Read the model definition and answer for the solid it produces. Units are mm, in the model's axes. A direction names the side the tool comes from. Coordinates: 2 decimals unless noted, no trailing zeros. Order: outer loops, then holes, each group sorted by start corner. A loop starts at its lowest first (then second) coordinate and runs counter-clockwise, first axis right, second up. Notation, with made-up numbers: (-6.5, -22) - (9.5, -22) arc R25 cw to (9.5, 6) - close; hole circle Ø11 at (-12, 2). An arc over 180 degrees is marked (long way). Use one line per item in the form item = value.
Autodesk Inventor part; units mm, degrees
ref_plane "YZ Plane" through (0, 0, 0) normal (1, 0, 0) x (0, 1, 0)
ref_plane "XZ Plane" through (0, 0, 0) normal (0, 1, 0) x (-1, 0, 0)
ref_plane "XY Plane" through (0, 0, 0) normal (0, 0, 1) x (1, 0, 0)
sketch "스케치6" plane through (0, 0, 0) normal (0, 1, 0) x (-1, 0, 0)
  circle A0 centre (0, 0) radius 15
  dimension "d16" = 30
extrude "돌출4" add sketch "스케치6" along normal blind 1.5
sketch "스케치7" plane through (0, 1.5, 0) normal (0, 1, 0) x (1, 0, 0)
  circle A0 centre (0, 0) radius 15
  arc A1 (0, 0) -> (-15, 0) centre (-7.5, -6.6144) ccw
  arc A2 (0, 0) -> (0, 15) centre (-6.6144, 7.5) ccw
  arc A3 (0, 0) -> (15, 0) centre (7.5, 6.6144) ccw
  arc A4 (0, 0) -> (0, -15) centre (6.6144, -7.5) ccw
  line L0 (0, -15) -> (0, 0)
  line L1 (0, 0) -> (15, 0)
  line L2 (0, 0) -> (0, 15)
  line L3 (0, 0) -> (-15, 0)
  arc A5 (-15, 0) -> (0, -15) centre (0, 0) ccw
  arc A6 (0, -15) -> (15, 0) centre (0, 0) ccw
  arc A7 (15, 0) -> (0, 15) centre (0, 0) ccw
  arc A8 (0, 15) -> (-15, 0) centre (0, 0) ccw
  point P0 (0, -15)
  point P1 (0, -15)
  dimension "d19" = 10
  dimension "d20" = 10
  dimension "d21" = 10
  dimension "d22" = 10
  dimension "d23" = 15
  dimension "d24" = 15
extrude "돌출5" cut sketch "스케치7" against normal blind 1.5 contours L1 A2 A0 | A0 L0 A3 | L2 A1 A0 | A0 L3 A4
sketch "스케치8" plane through (0, 1.5, 0) normal (0, 1, 0) x (1, 0, 0)
  arc A0 (0, 0) -> (0, -15) centre (6.6144, -7.5) ccw
  circle A1 centre (0, 0) radius 0.75
  dimension "d27" = 1.5
extrude "돌출6" add sketch "스케치8" against normal blind 1.5
sketch "스케치9" plane through (0, 1.5, 0) normal (0, 1, 0) x (1, 0, 0)
  point P0 (0, 0)
properties part number "fan_num4_1"
(1) Given pin 1 Ø0.8 at (x, y) = (6.5, 0.5) entering from -Z; pin 2 Ø0.8 at (y, z) = (1, 9) entering from +X, each flat-ended and moving along its own axis, determine where each tip first touches the part or whether it passes through.
Answer list:
pin_1 = 0
pin_2 = 0
(2) The mould has two halves that part along Z. Classify faces 5 (the cylindrical face through (-3.382, 0.76, 7.762)), 6 (the cylindrical face through (7.762, 0.76, 3.382)), 7 (the flat face through (0, 0, 0)): +Z half, -Z half, draft (parallel to the pull), parting line (faces both ways), or undercut.
Answer list:
face_5 = undercut
face_6 = +Z half
face_7 = draft
(3) Section B-B, the plane z = 1.25 is taken. Write down the section's boundary in (x, y).
Answer list:
outline = (-1.19, 0) - (0, 0) - (0, 1.5) - (-1.19, 1.5) - close; (1.32, 0) - (13.68, 0) - (13.68, 1.5) - (1.32, 1.5) - close
(4) Straight lines are drawn through the part: L1, parallel to Z at x = -1.5, y = 0.7; L2, parallel to Z at x = 7.25, y = 1.45; L3, parallel to X at y = 0.85, z = 12. For each, find the intervals that lie inside material, in ascending order.
Answer list:
L1 = -1.39 to 0, 1.66 to 13.34
L2 = 0 to 3.38
L3 = -2.32 to 0
(5) Which of the six approach directions +Z, -Z, +X, -X, +Y, -Y give full straight-line access (tool end or side, diameter ignored) to faces 1 (the flat face through (-8, 1, 0)), 2 (the flat face through (0, 1, -8)), 3 (the flat face through (0, 1, 8)), 4 (the flat face through (8, 1, 0))?
Answer list:
face_1 = -X, +Y, -Y
face_2 = -Z, +Y, -Y
face_3 = +Z, +Y, -Y
face_4 = +X, +Y, -Y
(6) Section A-A, the plane y = 0.8 is taken. Write down the section's boundary in (x, z), then the cut area to 3 significant figures.
Answer list:
outline = (-15, 0) arc R10 ccw to (-0.52, -0.54) arc R0.75 ccw to (0, -0.75) - (0, -15) arc R10 ccw to (0.54, -0.52) arc R0.75 ccw to (0.75, 0) - (15, 0) arc R10 ccw to (0.52, 0.54) arc R0.75 ccw to (0, 0.75) - (0, 15) arc R10 ccw to (-0.54, 0.52) arc R0.75 ccw to (-0.75, 0) - close
area = 142 mm2
(7) Section C-C, the plane x = 13.25 is taken. Write down the section's boundary in (y, z).
Answer list:
outline = (0, 0) - (1.5, 0) - (1.5, 1.57) - (0, 1.57) - close
(8) Section D-D, the plane z = 9.5 is taken. Write down the section's boundary in (x, y).
Answer list:
outline = (-3.18, 0) - (0, 0) - (0, 1.5) - (-3.18, 1.5) - close
